Could you check a few things on this model? Use its own coordinates, in mm. A direction names the side the tool comes from. Give positions to 0.01 mm unless a question says otherwise; leave off trailing zeros. Write each loop counter-clockwise with the first axis right and the second up, starting at its lowest first coordinate (ties: lowest second). Pieces come first, ordered by that corner, then holes. Notation, with made-up numbers: (69.25, 24.5) - (98.25, 24.5) arc R21 ccw to (98.25, 40.5) - close; hole circle Ø6 at (-25, 44). An arc over 180 degrees is marked (long way). Answer as a JSON object with one key per item and string values. Group by question number.
```python
from build123d import *
from build123d.topology import SkipClean

# Parameters (mm, degrees)
SKETCH2_R                = 44.5
BOSS_EXTRUDE1_DEPTH      = 93
BOSS_EXTRUDE2_START      = -30
SKETCH2_3_R              = 12.5
BOSS_EXTRUDE2_DEPTH      = 62
EXTRUDE_THIN1_DEPTH      = 115
CUT_EXTRUDE1_START       = -30
CUT_EXTRUDE1_OUTLINE_R   = 8.5
CUT_EXTRUDE1_OUTLINE_R_2 = 40.5
CUT_EXTRUDE1_DEPTH       = 123
RIB1_START               = -2.5
RIB1_DEPTH               = 5
FILLET1_R                = 10


# Read off the part's stored shape, not the designer's step: Cut-Extrude1, Rib1
with BuildPart() as part:
    # Sketch2 → Boss-Extrude1 (new body)
    with BuildSketch(Plane(origin=(0, 0, 0), x_dir=(1, 0, 0), z_dir=(0, 1, 0))):
        with Locations(Location((0, 0, 0), (0, 0, 90))):
            Circle(SKETCH2_R)
    extrude(amount=BOSS_EXTRUDE1_DEPTH)



with BuildPart() as body_2:
    # Sketch2<3> → Boss-Extrude2 (new body)
    with BuildSketch(Plane(origin=(0, 0, 0), x_dir=(1, 0, 0), z_dir=(0, 1, 0)).offset(BOSS_EXTRUDE2_START)):
        with Locations(Location((178, 0, 0), (0, 0, 270))):
            Circle(SKETCH2_3_R)
    extrude(amount=BOSS_EXTRUDE2_DEPTH)


with BuildPart() as part_1:
    add(part.part)

    add(body_2.part)  # Extrude-Thin1 merges body 2
    # Sketch3 → Extrude-Thin1 (add, symmetric)
    with BuildSketch(Plane.XY):
        Polygon((-44.5, 0), (102.247392222, 0), (138, -30), (190.5, -30), (190.5, -24), (140.183821406, -24), (104.431213628, 6), (-44.5, 6), align=None)
    extrude(amount=EXTRUDE_THIN1_DEPTH, both=True)

    # Cut-Extrude1 outline → Cut-Extrude1 (cut)
    with SkipClean():  # the faces are left unmerged after this step: merging them gives an invalid solid
        with BuildSketch(Plane(origin=(0, 0, 0), x_dir=(1, 0, 0), z_dir=(0, 1, 0)).offset(CUT_EXTRUDE1_START)):
            with Locations((178, 0)):
                Circle(CUT_EXTRUDE1_OUTLINE_R)
            with BuildLine():
                ThreePointArc((-44.5, 0), (-28.497806933, 34.1778437), (8, 43.774992861))
                Line((8, 43.774992861), (180.247191011, 12.296346309))
                ThreePointArc((180.247191011, 12.296346309), (187.600517893, 8.005001948), (190.5, 0))
                Line((190.5, 0), (190.5, 115))
                Line((190.5, 115), (-44.5, 115))
                Line((-44.5, 115), (-44.5, 0))
            make_face()
            with BuildLine():
                ThreePointArc((8, -43.774992861), (-28.497806933, -34.1778437), (-44.5, 0))
                Line((-44.5, 0), (-44.5, -115))
                Line((-44.5, -115), (190.5, -115))
                Line((190.5, -115), (190.5, 0))
                ThreePointArc((190.5, 0), (187.600517893, -8.005001948), (180.247191011, -12.296346309))
                Line((180.247191011, -12.296346309), (8, -43.774992861))
            make_face()
            Circle(CUT_EXTRUDE1_OUTLINE_R_2)
        extrude(amount=CUT_EXTRUDE1_DEPTH, mode=Mode.SUBTRACT)

    # Rib1 outline → Rib1 (add)
    with BuildSketch(Plane.XY.offset(RIB1_START)):
        Polygon((160.566154525, 32), (87.869185376, 93), (43, 93), (43, 6), (104.431213628, 6), (140.183821406, -24), (167, -24), (167, 32), align=None)
    extrude(amount=RIB1_DEPTH)

    # Fillet1
    fillet1_edges = [part_1.edges().sort_by_distance(p)[0] for p in [
        (140.183821406, -24, -11.05901849),
        (104.431213628, 6, -14.325962052),
        (160.566154525, 32, 0),
        (87.869185376, 93, 0),
        (102.247392222, 0, 0),
        (104.431213628, 6, 14.325962052),
        (140.183821406, -24, 11.05901849),
        (138, -30, 0),
    ]]
    fillet(fillet1_edges, radius=FILLET1_R)


solid = part_1.part
```
(1) I want a section at A-A, the plane y = 22. Please give me the cut outline in (x, z).
(2) Will these pins go through, and if not, where does the flat tip stop? P1, Ø5, axis at x = 161, z = 6, coming from the +Y side; P2, Ø7.5, axis at x = 173, z = 1, coming from the +Y side; P3, Ø4, axis at x = 78, y = 21, coming from the -Z side.
(3) If we mould it in two halves opening along Z, with no side actions, what happens to faces 1 (the flat face through (104, 35, -2.5)), 2 (the cylindrical face through (138.17, -29.38, 0.29)), 3 (the cylindrical face through (169.51, 0.57, -0.37))? For each: +Z half, -Z half, draft (parallel to the pull), parting line (faces both ways), or undercut.
(4) I want a section at D-D, the plane y = -16.5. Please give me the cut outline in (x, z), and give its area (3 significant figures).
(5) I want a section at B-B, the plane z = 31.5. Please give me the cut outline in (x, y).
(6) I want a section at C-C, the plane x = 79. Please give me the cut outline in (y, z), and give its area (3 significant figures).
(7) I need wall thicknesses on L1, parallel to X at y = 9, z = 0; L2, parallel to X at y = 9, z = 11; L3, parallel to Y at x = 57.5, z = 8. Which ranges of each line are inside material? Lowest first, please.
(8) For faces 4 (the flat face through (158, -24, 11)), 5 (the flat face through (186.3, 32, 2.6)), 6 (the flat face through (122.52, -9.18, -11.34)), which set-ups out of +Z, -Z, +X, -X, +Y, -Y let a thin tool reach every point of the face, with its end or its side?
Entries:
{
 "1": {"outline": "(44.43, -2.5) - (165.75, -2.5) arc R12.5 ccw (long way) to (165.75, 2.5) - (44.43, 2.5) arc R44.5 ccw (long way) to start; hole circle Ø81 at (0, 0); hole circle Ø17 at (178, 0)"},
 "2": {"P1": "y = -24", "P2": "y = 32", "P3": "z = -2.5"},
 "3": {"face 1": "-Z half", "face 2": "draft", "face 3": "undercut"},
 "4": {"outline": "(121.91, -22.96) - (131.25, -21.25) - (131.25, -2.5) - (165.75, -2.5) arc R12.5 ccw (long way) to (165.75, 2.5) - (131.25, 2.5) - (131.25, 21.25) - (121.91, 22.96) - close; hole circle Ø17 at (178, 0)", "area": "848 mm^2"},
 "5": {"outline": "(-31.43, 0) - (-25.46, 0) - (-25.46, 93) - (-31.43, 93) - close; (25.46, 0) - (75.17, 0) - (75.17, 6) - (31.43, 6) - (31.43, 93) - (25.46, 93) - close"},
 "6": {"outline": "(0, -30.8) - (6, -30.8) - (6, -2.5) - (93, -2.5) - (93, 2.5) - (6, 2.5) - (6, 30.8) - (0, 30.8) - close", "area": "805 mm^2"},
 "7": {"L1": "-44.5 to -40.5, 40.5 to 169.5, 186.5 to 190.5", "L2": "-43.12 to -38.98, 38.98 to 43.12, 172.06 to 183.94", "L3": "0 to 6"},
 "8": {"face 4": "+Z, +Y", "face 5": "+Z, -Z, +X, +Y", "face 6": "-Z, +Y"}
}
